Can you work these out from the drawing? Everything is in mm from the part's minimum corner. Round coordinates to 2 decimals unless told otherwise and drop trailing zeros. Write each loop counter-clockwise with the first axis right and the second up, starting at its lowest first coordinate (ties: lowest second). Pieces come first, ordered by that corner, then holes. Notation, with made-up numbers: M -35.75,17 L 21.25,17 A35 ccw 21.25,55 Z; hole C -14,-3.5 d5. An arc over 180 degrees is marked long. Use one line per item in the form item = value. Start each with the question number.
Q1. I'm going to push flat-ended pins straight in: pin 1 Ø0.6 at (y, z) = (28, 0.5) entering from -X; pin 2 Ø0.6 at (x, z) = (2, 0.5) entering from +Y; pin 3 Ø0.6 at (y, z) = (1.5, 1) entering from +X. Where does each tip first touch, or does it pass through?
Q2. I want a section at B-B on x = 31.85. List the corners of the cut face in (y, z) for me, and give its area (3 significant figures).
Q3. I want a section at A-A on y = 14.5. List the corners of the cut face in (x, z) for me.
Q4. I need wall thicknesses on line 1 along Y through (x, z) = (31.85, 1.4); line 2 along Y through (x, z) = (11.25, 0.6); line 3 along Y through (x, z) = (30.5, 0.85). Which ranges of each line are inside material? Lowest first, please. Write a range as from..to.
Q5. I want a section at D-D on x = 11.25. List the corners of the cut face in (y, z) for me, and give its area (3 significant figures).
Q6. I want a section at C-C on z = 0.9. List the corners of the cut face in (x, y) for me.
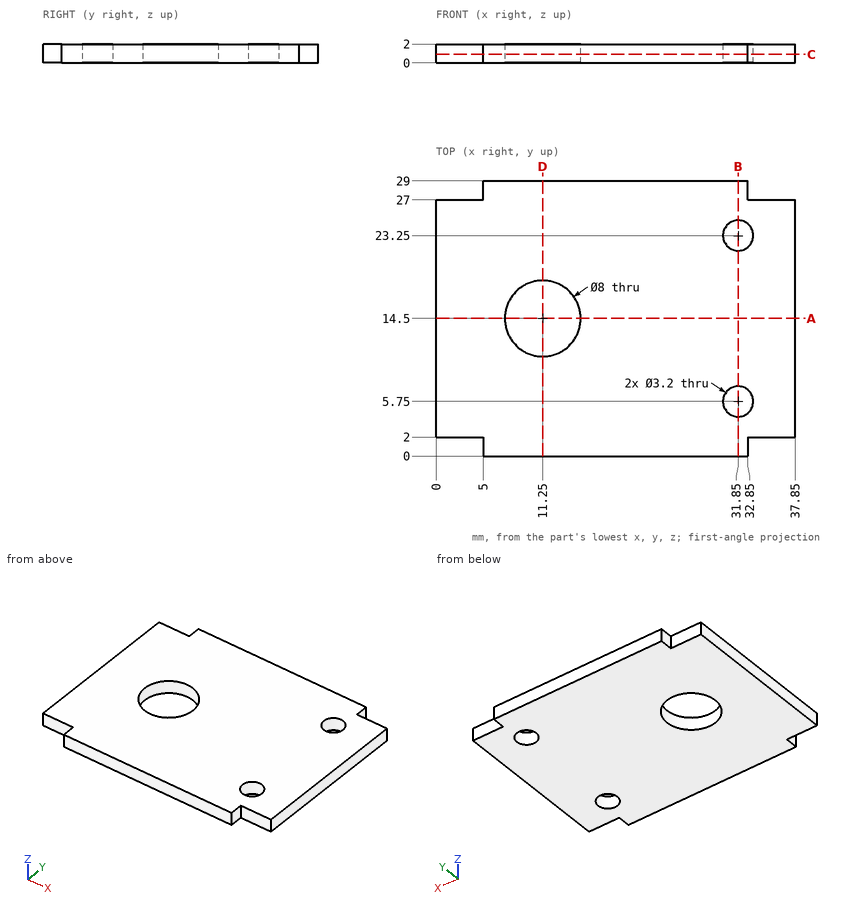
Reported:
q1.pin_1 = 5
q1.pin_2 = 27
q1.pin_3 = 32.85
q2.outline = M 0,0 L 4.15,0 L 4.15,2 L 0,2 Z; M 7.35,0 L 21.65,0 L 21.65,2 L 7.35,2 Z; M 24.85,0 L 29,0 L 29,2 L 24.85,2 Z
q2.area = 45.2 mm^2
q3.outline = M 0,0 L 7.25,0 L 7.25,2 L 0,2 Z; M 15.25,0 L 37.85,0 L 37.85,2 L 15.25,2 Z
q4.line_1 = 0..4.15, 7.35..21.65, 24.85..29
q4.line_2 = 0..10.5, 18.5..29
q4.line_3 = 0..4.89, 6.61..22.39, 24.11..29
q5.outline = M 0,0 L 10.5,0 L 10.5,2 L 0,2 Z; M 18.5,0 L 29,0 L 29,2 L 18.5,2 Z
q5.area = 42.0 mm^2
q6.outline = M 0,2 L 5,2 L 5,0 L 32.85,0 L 32.85,2 L 37.85,2 L 37.85,27 L 32.85,27 L 32.85,29 L 5,29 L 5,27 L 0,27 Z; hole C 11.25,14.5 d8; hole C 31.85,5.75 d3.2; hole C 31.85,23.25 d3.2
